Check sheet for the modelled part. Datum: model origin and axes. Units: mm. Coordinates: 2 decimals unless noted, no trailing zeros. Order: outer loops, then holes, each group sorted by start corner. A loop starts at its lowest first (then second) coordinate and runs counter-clockwise, first axis right, second up.
1. Cross-section at A-A (y = 0.5). Enter the section's corners in (x, z), then the cut area to 4 significant figures.
2. Thickness scan on line 1 (X direction, y = -2.5, z = -1.3); line 2 (Y direction, x = -11.5, z = 0.2); line 3 (Y direction, x = 2.5, z = 1.6). Record the ranges inside material, lowest first.
3. Gauge pin test, flat end, axial feed: pin 1 Ø2.5 at (x, y) = (-7.5, 0.5) entering from +Z. Record the tip position at first contact, or that the pin passes through.
4. Cross-section at B-B (x = 19). Enter the section's corners in (y, z), then the cut area to 3 significant figures.
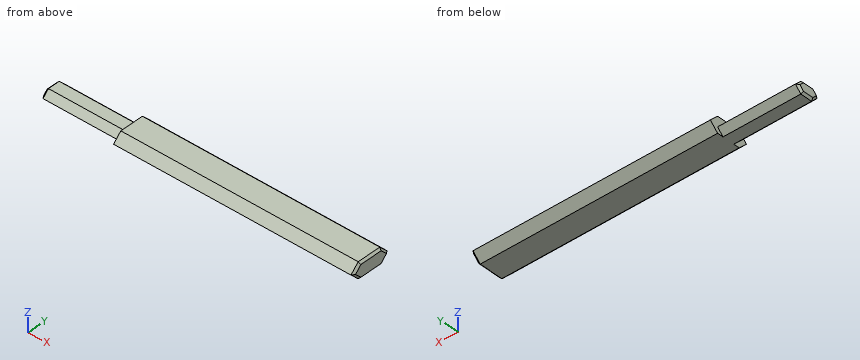
Autodesk Fusion 360 part; units mm, degrees
sketch "Sketch1" plane through (0, 0, 0) normal (1, 0, 0) x (0, 1, 0)
  line L0 (-3, 2) -> (3, 2)
  line L1 (3, 2) -> (3, -2)
  line L2 (3, -2) -> (-3, -2)
  line L3 (-3, -2) -> (-3, 2)
  line L4 (3, 2) -> (5, 0)
  line L5 (5, 0) -> (3, -2)
  line L6 (-3, 2) -> (-5, 0)
  line L7 (-5, 0) -> (-3, -2)
  line L8 (-3, 2) -> (3, -2) construction
  line L9 (3, 2) -> (-3, -2) construction
  dimension "d1" = 10
  dimension "d2" = 2
  dimension "d3" = 4
extrude "Extrude1" add sketch "Sketch1" along normal blind 60
sketch "Sketch2" plane through (0, 0, 0) normal (-1, 0, 0) x (0, -1, 0)
  line L0 (5, 0) -> (3, 2)
  line L1 (-3, 2) -> (-5, 0)
  line L2 (-5, 0) -> (-3, -2)
  line L3 (3, -2) -> (5, 0)
  line L4 (-1.5, 1) -> (1.5, 1)
  line L5 (1.5, 1) -> (1.5, -2)
  line L6 (1.5, -2) -> (-1.5, -2)
  line L7 (-1.5, -2) -> (-1.5, 1)
  line L8 (1.5, 1) -> (3, -0.5)
  line L9 (3, -0.5) -> (1.5, -2)
  line L10 (-1.5, 1) -> (-3, -0.5)
  line L11 (-3, -0.5) -> (-1.5, -2)
  line L12 (3, 2) -> (-3, 2)
  dimension "d12" = 3
  dimension "d13" = 1.5
  dimension "d14" = 45
  dimension "d15" = 45
  dimension "d16" = 1
extrude "Extrude2" add sketch "Sketch2" along normal blind 20
chamfer "Chamfer1" distance 0.5 angle 45 1 faces at (60, -1, -0.6667)
chamfer "Chamfer3" distance 0.5 angle 45 1 faces at (-20, 0.5, 0)
equation "d13 = d12 / 2"
Data:
1. outline: (-20, -1.5) - (-19.5, -2) - (59.5, -2) - (60, -1.5) - (60, 1.5) - (59.5, 2) - (0, 2) - (0, 1) - (-19.5, 1) - (-20, 0.5) - close
1. area: 299.5 mm2
2. line 1: x = 0 to 60
2. line 2: y = -2.3 to 2.3
2. line 3: y = -3.4 to 3.4
3. pin 1: stops at z = 1
4. outline: (-5, 0) - (-3, -2) - (3, -2) - (5, 0) - (3, 2) - (-3, 2) - close
4. area: 32.0 mm2
